```python
from build123d import *

# Parameters (mm, degrees)
BOSS_EXTRUDE5_DEPTH = 50
BOSS_EXTRUDE6_DEPTH = 2


with BuildPart() as part:
    # Sketch1 → Boss-Extrude5 (new body)
    with BuildSketch(Plane(origin=(0, 0, 0), x_dir=(1, 0, 0), z_dir=(0, 1, 0))):
        Polygon((-148.684110885, 49.061860601), (-183.684110885, 29.061860601), (-183.684110885, -20.938139399), (-148.684110885, -40.938139399), (92.307295507, -20.938139399), (92.307295507, -14.938139399), (92.307295507, 23.061860601), (92.307295507, 29.061860601), align=None)
        Polygon((-177.684110885, -20.938139399), (-177.684110885, 29.061860601), (-148.684110885, 43.061860601), (86.307295507, 23.559803668), (86.307295507, 23.061860601), (86.307295507, -14.938139399), (86.307295507, -15.436082465), (-148.684110885, -34.938139399), align=None, mode=Mode.SUBTRACT)
    extrude(amount=BOSS_EXTRUDE5_DEPTH)

    # Sketch3 → Boss-Extrude6 (add)
    with BuildSketch(Plane.XZ):
        Polygon((-183.684110885, 20.938139399), (-183.684110885, -29.061860601), (-148.684110885, -49.061860601), (92.307295507, -29.061860601), (92.307295507, 20.938139399), (-148.684110885, 40.938139399), align=None)
    extrude(amount=BOSS_EXTRUDE6_DEPTH)


solid = part.part
```
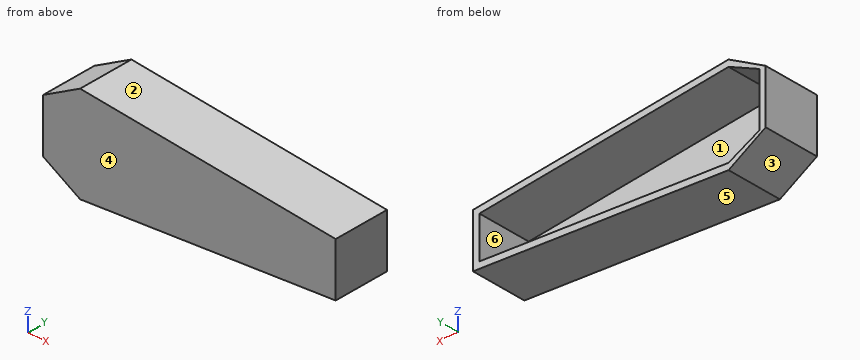
Here's how the part is built. I have some questions about the finished solid (model axes, mm). Face numbers are marked on the shaded views. A direction names the side the tool comes from. Coordinates: 2 decimals unless noted, no trailing zeros. Loops run counter-clockwise (first coordinate to the right, second up) from the corner with the lowest first, then second, coordinate; pieces in that order, holes last. Notation, with made-up numbers: (-7.5, 67) - (18.5, 67) arc R22 ccw to (18.5, 83) - close; hole circle Ø6 at (78, 45.5). An arc over 180 degrees is marked (long way). Return JSON: item names as keys, results as strings. Group by question number.
Item 1: We'd pull the mould along X, two halves only. Please class the marked faces 3, 4, 5 and 6: +X half, -X half, draft (parallel to the pull), parting line (faces both ways), or undercut.
Item 2: If we section it at C-C on z = -7.5: Write out the boundary of the cut face in (x, y), and give its area (3 significant figures).
Item 3: I need wall thicknesses on line 1 (X direction, y = 42, z = 3); line 2 (Y direction, x = -62, z = -26.5); line 3 (Z direction, x = -14, y = 11). Which ranges of each line are inside material? Lowest first, please. Write a range as from..to.
Item 4: If we section it at A-A on y = 14: Write out the boundary of the cut face in (x, z), and give its area (3 significant figures).
Item 5: If we section it at B-B on x = 6: Write out the boundary of the cut face in (y, z).
Item 6: Will these pins go through, and if not, where does the flat tip stop? P1, Ø2, axis at x = 30.5, y = 37, coming from the -Z side; P2, Ø4, axis at x = -52, y = 18, coming from the +Z side; P3, Ø1.5, axis at x = 23, z = -3.5, coming from the +Y side.
Item 7: On a 3-axis mill with a long thin cutter (end or side, diameter ignored), from which of +Z, -Z, +X, -X, +Y, -Y can I reach the whole of each face in a straight line? I mean the marked faces 1 and 2. Say none if no direction works.
Calculated:
{
 "1": {"face 3": "-X half", "face 4": "draft", "face 5": "+X half", "face 6": "undercut"},
 "2": {"outline": "(-183.68, -2) - (92.31, -2) - (92.31, 50) - (86.31, 50) - (86.31, 0) - (-177.68, 0) - (-177.68, 50) - (-183.68, 50) - close", "area": "1,150 mm^2"},
 "3": {"line 1": "x = -183.68..-177.68, 86.31..92.31", "line 2": "y = -2..0", "line 3": "z = -37.88..-31.88, 23.76..29.76"},
 "4": {"outline": "(-183.68, -29.06) - (-148.68, -49.06) - (92.31, -29.06) - (92.31, 20.94) - (-148.68, 40.94) - (-183.68, 20.94) - close; hole (-177.68, -29.06) - (-148.68, -43.06) - (86.31, -23.56) - (86.31, 15.44) - (-148.68, 34.94) - (-177.68, 20.94) - close", "area": "3,720 mm^2"},
 "5": {"outline": "(-2, -36.22) - (50, -36.22) - (50, -30.22) - (0, -30.22) - (0, 22.1) - (50, 22.1) - (50, 28.1) - (-2, 28.1) - close"},
 "6": {"P1": "stops at z = -34.27", "P2": "stops at z = 33.08", "P3": "stops at y = 0"},
 "7": {"face 1": "+Y", "face 2": "+Z, +X, +Y, -Y"}
}
